from build123d import *
from build123d.topology import SkipClean

# Parameters (mm, degrees)
EXTRUDE_1_DEPTH     = 3
SKETCH_2_R          = 1.5
CUT_EXTRUDE_1_DEPTH = 3
EXTRUDE_2_DEPTH     = 3
FILLET_1_R          = 1
FILLET_2_R          = 1
CUT_EXTRUDE_2_DEPTH = 3
EXTRUDE_START       = -17.477520588
EXTRUDE_3_DEPTH     = 20.477520588
EXTRUDE_START_2     = -11.853392215
EXTRUDE_3_2_DEPTH   = 23.70678443
EXTRUDE_4_REACH     = 165.663
SKETCH_6_W          = 66
SKETCH_6_H          = 4
EXTRUDE_6_REACH     = 172.329
EXTRUDE_7_REACH     = 172.329
CUT_EXTRUDE_3_DEPTH = 4


with BuildPart() as part:
    # 草图1 → 凸台-拉伸1 (new body)
    with BuildSketch(Plane(origin=(0, 0, 0), x_dir=(1, 0, 0), z_dir=(0, 1, 0))):
        Polygon((25, 11.878712678), (25, -11.878712678), (130, -9.252891981), (130, 9.252891981), align=None)
    extrude(amount=EXTRUDE_1_DEPTH)

    # 草图2 → 切除-拉伸1 (cut)
    with BuildSketch(Plane(origin=(0, 3, 0), x_dir=(1, 0, 0), z_dir=(0, 1, 0))):
        with Locations(Location((37, 8, 0), (0, 0, 270))):
            Circle(SKETCH_2_R)
        with Locations(Location((37, -8, 0), (0, 0, 270))):
            Circle(SKETCH_2_R)
        with Locations(Location((87, 0, 0), (0, 0, 270))):
            Circle(SKETCH_2_R)
    extrude(amount=-CUT_EXTRUDE_1_DEPTH, mode=Mode.SUBTRACT)

    # 草图3 → 凸台-拉伸2 (add)
    with BuildSketch(Plane(origin=(0, 3, 0), x_dir=(1, 0, 0), z_dir=(0, 1, 0))):
        Polygon((33, 5.676774269), (33, 7.677399562), (31, 7.727415195), (31, 5.726789902), align=None)
        Polygon((33, 0), (33, 5.676774269), (31, 5.726789902), (31, 0), align=None)
        Polygon((33, -5.676774269), (33, 0), (31, 0), (31, -5.726789902), align=None)
        Polygon((33, -7.677399562), (33, -5.676774269), (31, -5.726789902), (31, -7.727415195), align=None)
        Polygon((43, 7.427321401), (41, 7.477337033), (41, 5.47671174), (43, 5.426696108), align=None)
        Polygon((43, 5.426696108), (41, 5.47671174), (41, 0), (43, 0), align=None)
        Polygon((43, 0), (41, 0), (41, -5.47671174), (43, -5.426696108), align=None)
        Polygon((43, -5.426696108), (41, -5.47671174), (41, -7.477337033), (43, -7.427321401), align=None)
        Polygon((55.9, 7.104720572), (43, 7.427321401), (43, 5.426696108), (55.9, 5.104095279), align=None)
        Polygon((55.9, -5.104095279), (43, -5.426696108), (43, -7.427321401), (55.9, -7.104720572), align=None)
        Polygon((57.9, 7.05470494), (55.9, 7.104720572), (55.9, 5.104095279), (57.9, 5.054079647), align=None)
        Polygon((57.9, 5.054079647), (55.9, 5.104095279), (55.9, 0), (57.9, 0), align=None)
        Polygon((57.9, 0), (55.9, 0), (55.9, -5.104095279), (57.9, -5.054079647), align=None)
        Polygon((57.9, -5.054079647), (55.9, -5.104095279), (55.9, -7.104720572), (57.9, -7.05470494), align=None)
        Polygon((68.1, 6.799625215), (66.1, 6.849640847), (66.1, 4.849015554), (68.1, 4.798999922), align=None)
        Polygon((68.1, 4.798999922), (66.1, 4.849015554), (66.1, 0), (68.1, 0), align=None)
        Polygon((68.1, 0), (66.1, 0), (66.1, -4.849015554), (68.1, -4.798999922), align=None)
        Polygon((68.1, -4.798999922), (66.1, -4.849015554), (66.1, -6.849640847), (68.1, -6.799625215), align=None)
        Polygon((81, 6.477024386), (68.1, 6.799625215), (68.1, 4.798999922), (81, 4.476399093), align=None)
        Polygon((81, -4.476399093), (68.1, -4.798999922), (68.1, -6.799625215), (81, -6.477024386), align=None)
        Polygon((83, -4.426383461), (81, -4.476399093), (81, -6.477024386), (83, -6.427008754), align=None)
        Polygon((83, 0), (81, 0), (81, -4.476399093), (83, -4.426383461), align=None)
        Polygon((83, 4.426383461), (81, 4.476399093), (81, 0), (83, 0), align=None)
        Polygon((83, 6.427008754), (81, 6.477024386), (81, 4.476399093), (83, 4.426383461), align=None)
        Polygon((93, 6.176930593), (91, 6.226946225), (91, 4.226320932), (93, 4.176305299), align=None)
        Polygon((93, 4.176305299), (91, 4.226320932), (91, 0), (93, 0), align=None)
        Polygon((93, 0), (91, 0), (91, -4.226320932), (93, -4.176305299), align=None)
        Polygon((93, -4.176305299), (91, -4.226320932), (91, -6.226946225), (93, -6.176930593), align=None)
    extrude(amount=EXTRUDE_2_DEPTH)

    # 圆角1
    fillet_1_edges = [part.edges().sort_by_distance(p)[0] for p in [
        (91, 4.5, -6.226946225),
        (91, 4.5, 6.226946225),
        (93, 4.5, 6.176930593),
        (93, 4.5, -6.176930593),
        (31, 4.5, -7.727415195),
        (31, 4.5, 7.727415195),
        (33, 4.5, 7.677399562),
        (33, 4.5, -7.677399562),
        (41, 4.5, 7.477337033),
        (57.9, 4.5, 7.05470494),
        (57.9, 4.5, -7.05470494),
        (41, 4.5, -7.477337033),
        (66.1, 4.5, 6.849640847),
        (83, 4.5, 6.427008754),
        (83, 4.5, -6.427008754),
        (66.1, 4.5, -6.849640847),
    ]]
    fillet(fillet_1_edges, radius=FILLET_1_R - 0.0001)  # a hair under: the kernel refuses the full size

    # 圆角2
    fillet_2_edges = [part.edges().sort_by_distance(p)[0] for p in [
        (25, 1.5, 11.878712678),
        (25, 1.5, -11.878712678),
    ]]
    fillet(fillet_2_edges, radius=FILLET_2_R)

    # 草图4 → 切除-拉伸2 (cut)
    with BuildSketch(Plane(origin=(0, 3, 0), x_dir=(1, 0, 0), z_dir=(0, 1, 0))):
        Polygon((43, 5.426696108), (55.9, 5.104095279), (55.9, -5.104095279), (43, -5.426696108), align=None)
        Polygon((68.1, 4.798999922), (81, 4.476399093), (81, -4.476399093), (68.1, -4.798999922), align=None)
    extrude(amount=-CUT_EXTRUDE_2_DEPTH, mode=Mode.SUBTRACT)

    # 凸台-拉伸3: read off the stored shape, not the designer's step
    # 凸台-拉伸3 outline → 凸台-拉伸3 (add)
    with BuildSketch(Plane(origin=(0, 0, 0), x_dir=(1, 0, 0), z_dir=(0, 1, 0)).offset(EXTRUDE_START)):
        Polygon((130, -9.25289198), (160.262492185, -8.496093139), (160.262492185, 8.496093139), (130, 9.25289198), align=None)
    extrude(amount=EXTRUDE_3_DEPTH)

    # Extrude 3 2 outline → Extrude 3 2 (cut)
    with BuildSketch(Plane.XY.offset(EXTRUDE_START_2)):
        Polygon((130, 3), (160.262492185, -14.477520588), (160.262492185, 3), align=None)
        Polygon((160.262492185, -17.477520588), (130, 0), (130, -17.477520588), align=None)
    extrude(amount=EXTRUDE_3_2_DEPTH, mode=Mode.SUBTRACT)

    # 草图6 → 凸台-拉伸4 (add, up to next)
    with BuildSketch(Plane(origin=(0, -25, 0), x_dir=(-1, 0, 0), z_dir=(0, -1, 0)), mode=Mode.PRIVATE) as extrude_4_sk1:
        with Locations((-127.262492185, 0)):
            Rectangle(SKETCH_6_W, SKETCH_6_H)
    extrude_4_tool1 = extrude(extrude_4_sk1.sketch, amount=-EXTRUDE_4_REACH, mode=Mode.PRIVATE) - part.part
    add(extrude_4_tool1.solids().sort_by_distance((127.262492, -25, 0))[0])

    # 镜向21: part across plane


with BuildPart() as part_1:
    add(part.part)
    add(part.part.mirror(Plane(origin=(0, -25, 0), x_dir=(0, 0, 1), z_dir=(0, -1, 0))))

    # 凸台-拉伸6: up to this plane
    extrude_6_end = Plane(origin=(0.3125, 3, -12.496093139), z_dir=(0.024999999999999984, 0, -0.9996874511566103))
    # 草图8 → 凸台-拉伸6 (add, up to the surface)
    with BuildSketch(Plane(origin=(0, 0, -2), x_dir=(-1, 0, 0), z_dir=(0, 0, -1)), mode=Mode.PRIVATE) as extrude_6_sk1:
        Polygon((-160.262492185, -17.477520588), (-160.262492185, -32.522479412), (-156.262492185, -34.832602515), (-156.262492185, -15.167397485), align=None)
    extrude_6_tool1 = split(extrude(extrude_6_sk1.sketch, amount=EXTRUDE_6_REACH, mode=Mode.PRIVATE), bisect_by=extrude_6_end, keep=Keep.BOTH, mode=Mode.PRIVATE)
    add(extrude_6_tool1.solids().sort_by_distance((158.173753, -25, -2))[0])

    # 凸台-拉伸7: up to this plane
    extrude_7_end = Plane(origin=(0.3125, 3, 12.496093139), z_dir=(-0.024999999999999984, 0, -0.9996874511566103))
    # 草图9 → 凸台-拉伸7 (add, up to the surface)
    with BuildSketch(Plane.XY.offset(2), mode=Mode.PRIVATE) as extrude_7_sk1:
        Polygon((160.262492185, -17.477520588), (156.262492185, -15.167397485), (156.262492185, -34.832602515), (160.262492185, -32.522479412), align=None)
    extrude_7_tool1 = split(extrude(extrude_7_sk1.sketch, amount=EXTRUDE_7_REACH, mode=Mode.PRIVATE), bisect_by=extrude_7_end, keep=Keep.BOTH, mode=Mode.PRIVATE)
    add(extrude_7_tool1.solids().sort_by_distance((158.173753, -25, 2))[0])

    # 草图10 → 切除-拉伸3 (cut)
    with BuildSketch(Plane(origin=(0, 0, -2), x_dir=(-1, 0, 0), z_dir=(0, 0, -1))):
        Polygon((-142.327118039, -11.738453253), (-152.262492185, -17.476437591), (-152.262492185, -23), (-135.82322821, -23), align=None)
        Polygon((-135.82322821, -27), (-152.262492185, -27), (-152.262492185, -32.523562409), (-142.327118039, -38.261546747), align=None)
        Polygon((-128.927913048, -4), (-138.863287194, -9.737984338), (-131.204065001, -23), (-128.927913048, -23), align=None)
        Polygon((-128.927913048, -27), (-131.204065001, -27), (-138.863287194, -40.262015662), (-128.927913048, -46), align=None)
        Polygon((-101.09091931, -4), (-124.927913048, -4), (-124.927913048, -23), (-120.09091931, -23), align=None)
        Polygon((-120.09091931, -27), (-124.927913048, -27), (-124.927913048, -46), (-101.09091931, -46), align=None)
        Polygon((-98.262492185, -6.828427125), (-114.43406506, -23), (-114.43406506, -27), (-98.262492185, -43.171572875), align=None)
    extrude(amount=-CUT_EXTRUDE_3_DEPTH, mode=Mode.SUBTRACT)

    # 草图11 → 旋转1 (revolve)
    with SkipClean():  # the faces are left unmerged after this step: merging them gives an invalid solid
        with BuildSketch(Plane.XY, mode=Mode.PRIVATE) as revolve_1_sk:
            with BuildLine():
                Line((160.262492185, -25), (160.262492185, -32))
                ThreePointArc((160.262492185, -32), (165.212239653, -29.949747468), (167.262492185, -25))
                Line((167.262492185, -25), (160.262492185, -25))
            make_face()
            with BuildLine():
                Line((160.262492185, -18), (160.262492185, -25))
                Line((160.262492185, -25), (167.262492185, -25))
                ThreePointArc((167.262492185, -25), (165.212239653, -20.050252532), (160.262492185, -18))
            make_face()
        revolve(revolve_1_sk.sketch.rotate(Axis((160.262492185, -25, 0), (1, 0, 0)), 180), axis=Axis((160.262492185, -25, 0), (1, 0, 0)))
    add(part_1.part.scale(1), mode=Mode.REPLACE)  # the faces are merged on a copy


solid = part_1.part
Model file for the job. Use its own axes, mm. A direction names the side the tool comes from. Give positions to 0.01 mm unless a question says otherwise; leave off trailing zeros. Loops run counter-clockwise (first coordinate to the right, second up) from the corner with the lowest first, then second, coordinate; pieces in that order, holes last.
1) Tool access for faces 1 (the flat face through (119, -25, 2)), 2 (the flat face through (139.12, -32.71, -0.03)), 3 (the flat face through (77, -50, 5)): list every direction of +Z, -Z, +X, -X, +Y, -Y with a clear straight run to the whole face (end or side of a thin tool).
2) Saw through at D-D (x = 37). Write the cut outline in (y, z), plus the area to 3 significant figures.
3) Saw through at B-B (z = 0). Count the separate pieces of the cut face and the enclosed holes in it, plus the area to 3 significant figures.
4) Saw through at C-C (x = 106). Write the cut outline in (y, z), plus the area to 3 significant figures.
5) Flat gauge pins, fed straight in: pin 1 Ø1.5 at (y, z) = (-55, -1) entering from +X; pin 2 Ø5 at (y, z) = (-48.5, -0.5) entering from +X; pin 3 Ø3.5 at (x, z) = (87, 0) entering from -Y. Where does each tip first touch, or does it go through?
6) Saw through at A-A (y = -21). Write the cut outline in (x, z), plus the area to 3 significant figures.
7) Wall check: line 1 (Y direction, x = 35.5, z = -2.5); line 2 (Y direction, x = 108, z = -1); line 3 (X direction, y = -22, z = 1.5). Give the ranges that are in metal, low to high.
8) Pull direction X, two halves, no side cores. Call faces 4 (the flat face through (93, -54, 0)), 5 (the flat face through (139.03, -17.45, -0.03)), 6 (the flat face through (77, 0, 5)), 7 (the flat face through (147.23, -14.57, -0.03)): +X half, -X half, draft (parallel to the pull), parting line (faces both ways), or undercut.
Answer block:
1. face 1: +Z, -X
1. face 2: +Z, -Z
1. face 3: -X
2. outline: (-53, -11.58) - (-50, -11.58) - (-50, -9.5) - (-53, -9.5) - close; (-53, -6.5) - (-50, -6.5) - (-50, 6.5) - (-53, 6.5) - close; (-53, 9.5) - (-50, 9.5) - (-50, 11.58) - (-53, 11.58) - close; (0, -11.58) - (3, -11.58) - (3, -9.5) - (0, -9.5) - close; (0, -6.5) - (3, -6.5) - (3, 6.5) - (0, 6.5) - close; (0, 9.5) - (3, 9.5) - (3, 11.58) - (0, 11.58) - close
2. area: 103 mm2
3. separate pieces: 7
3. enclosed holes: 7
3. area: 2,230 mm2
4. outline: (-53, -9.85) - (-50, -9.85) - (-50, -2) - (-46, -2) - (-46, 2) - (-50, 2) - (-50, 9.85) - (-53, 9.85) - close; (-41.09, -2) - (-35.43, -2) - (-35.43, 2) - (-41.09, 2) - close; (-14.57, -2) - (-8.91, -2) - (-8.91, 2) - (-14.57, 2) - close; (-4, -2) - (0, -2) - (0, -9.85) - (3, -9.85) - (3, 9.85) - (0, 9.85) - (0, 2) - (-4, 2) - close
4. area: 195 mm2
5. pin 1: stops at x = 93
5. pin 2: stops at x = 142.12
5. pin 3: stops at y = -53
6. outline: (94.26, -2) - (98.26, -2) - (98.26, 2) - (94.26, 2) - close; (112.43, -2) - (118.09, -2) - (118.09, 2) - (112.43, 2) - close; (124.93, -2) - (128.93, -2) - (128.93, 2) - (124.93, 2) - close; (132.36, -2) - (136.98, -2) - (136.98, 2) - (132.36, 2) - close; (152.26, -2) - (156.26, -2) - (156.26, -8.6) - (160.26, -8.5) - (160.26, -5.74) arc R5.74 ccw to (160.26, 5.74) - (160.26, 8.5) - (156.26, 8.6) - (156.26, 2) - (152.26, 2) - close
6. area: 209 mm2
7. line 1: y = -53 to -50, 0 to 3
7. line 2: y = -53 to -46, -39.09 to -33.43, -16.57 to -10.91, -4 to 3
7. line 3: x = 94.26 to 98.26, 113.43 to 119.09, 124.93 to 128.93, 131.78 to 136.4, 152.26 to 166.41
8. face 4: +X half
8. face 5: undercut
8. face 6: draft
8. face 7: undercut
